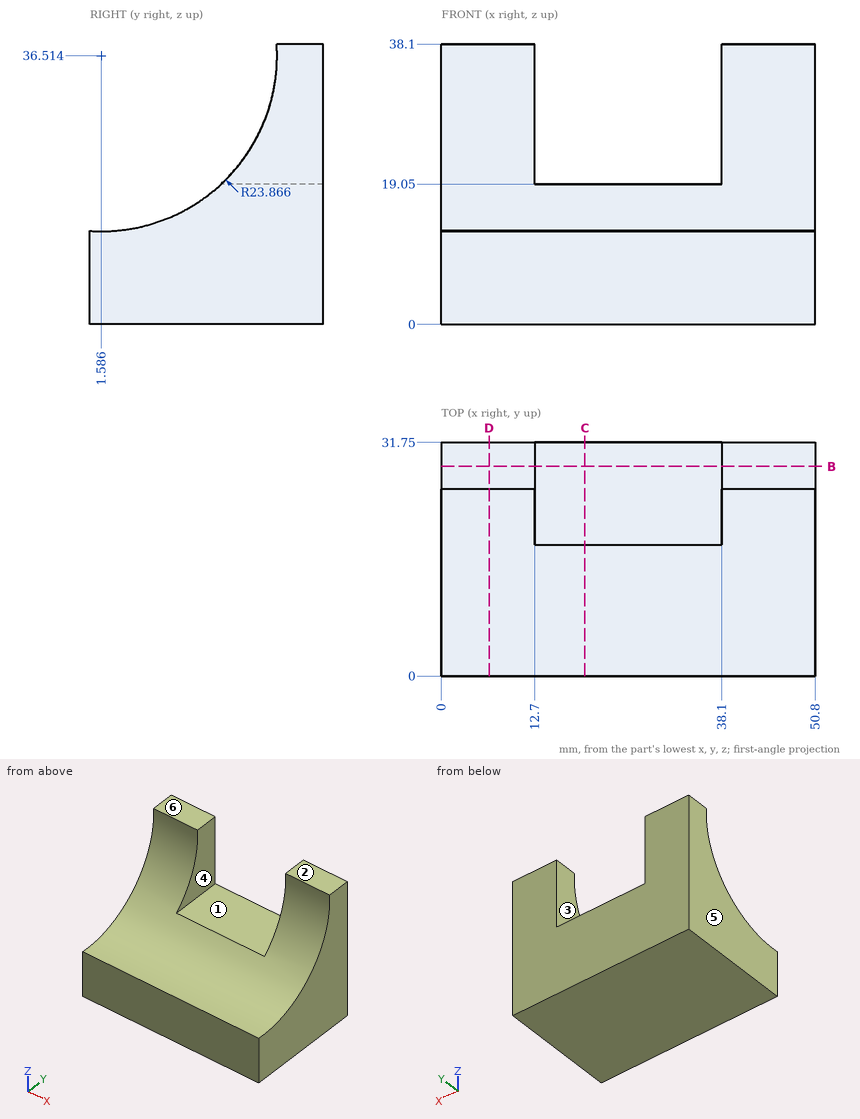
Part print with two shaded views. Sizes in mm from the minimum x, y, z corner. A direction names the side the tool comes from. Round coordinates to 2 decimals unless told otherwise and drop trailing zeros. Loops run counter-clockwise (first coordinate to the right, second up) from the corner with the lowest first, then second, coordinate; pieces in that order, holes last.
Item 1: Pin check, flat tips, straight feed: P1, Ø4, axis at y = 27.5, z = 24.5, coming from the -X side; P2, Ø7, axis at x = 31, y = 23, coming from the +Z side; P3, Ø5, axis at x = 17.5, y = 13, coming from the +Z side; P4, Ø12, axis at x = 9, y = 11, coming from the +Z side. Stop position of each tip, or through.
Item 2: Saw through at B-B (y = 28.5). List the corners of the cut face in (x, z).
Item 3: Saw through at C-C (x = 19.5). List the corners of the cut face in (y, z), then the cut area to 3 significant figures.
Item 4: Which spindle directions (+Z, -Z, +X, -X, +Y, -Y) get a long thin tool onto all of the face, cutting with end or side? Do the marked faces 1 and 2. Say none if no direction does.
Item 5: Saw through at D-D (x = 6.5). List the corners of the cut face in (y, z), then the cut area to 3 significant figures.
Item 6: Two-plate mould, pull along X, no slides. Class the marked faces 3, 4, 5 and 6: released by +X, released by -X, zero draft, split by the parting line, or undercut.
Item 7: Drill centre lines: line 1 along X through (y, z) = (26, 31.5); line 2 along Z through (x, y) = (14, 22); line 3 along Z through (x, y) = (19, 3). Where is each one in solid material? Low to high.
Worked answers:
1. P1: stops at x = 0
1. P2: stops at z = 19.05
1. P3: stops at z = 17.12
1. P4: stops at z = 18.29
2. outline: (0, 0) - (50.8, 0) - (50.8, 38.1) - (38.1, 38.1) - (38.1, 19.05) - (12.7, 19.05) - (12.7, 38.1) - (0, 38.1) - close
3. outline: (0, 0) - (31.75, 0) - (31.75, 19.05) - (17.85, 19.05) arc R23.87 cw to (0, 12.7) - close
3. area: 523 mm2
4. face 1: +Z, +Y, -Y
4. face 2: +Z, +X, -X, +Y, -Y
5. outline: (0, 0) - (31.75, 0) - (31.75, 38.1) - (25.4, 38.1) arc R23.87 cw to (0, 12.7) - close
5. area: 684 mm2
6. face 3: undercut
6. face 4: undercut
6. face 5: released by -X
6. face 6: zero draft
7. line 1: x = 0 to 12.7, 38.1 to 50.8
7. line 2: z = 0 to 19.05
7. line 3: z = 0 to 12.69
